Read the model definition and answer for the solid it produces. Units are mm, in the model's axes. Face numbers are marked on the shaded views. A direction names the side the tool comes from. Round coordinates to 2 decimals unless told otherwise and drop trailing zeros. Write each loop counter-clockwise with the first axis right and the second up, starting at its lowest first coordinate (ties: lowest second). Pieces come first, ordered by that corner, then holes. Notation, with made-up numbers: (73.5, -27.5) - (129.5, -27.5) arc R31 cw to (129.5, 0.5) - close; hole circle Ø9 at (29, 50). An arc over 180 degrees is marked (long way). One line per item, written item: value. Start each with the question number.
(1) A cutting plane is placed at A-A, the plane y = 3.5. Determine the outline of the cut face in (x, z), plus the area to 3 significant figures.
(2) For the marked faces 1 and 2, determine the directions among +Z, -Z, +X, -X, +Y, -Y from which every point of the face is accessible in a straight line to the end or side of a thin tool.
(3) Find the intervals of material crossed by L1, parallel to Y at x = 0, z = 0.85; L2, parallel to X at y = -3.5, z = 0.4; L3, parallel to Y at x = 10.25, z = 1.8, in increasing order.
(4) A cutting plane is placed at C-C, the plane y = -3.5. Determine the outline of the cut face in (x, z), plus the area to 3 significant figures.
(5) A cutting plane is placed at D-D, the plane z = 0.85. Determine the outline of the cut face in (x, y).
(6) Flat-ended cylindrical pins translate along their axes: pin 1 Ø1.8 at (x, y) = (7, 3.5) entering from -Z; pin 2 Ø1.5 at (x, y) = (6, 4.5) entering from +Z. Find the tip coordinate at first contact, or state that the pin passes through.
(7) A cutting plane is placed at B-B, the plane x = 0. Determine the outline of the cut face in (y, z).
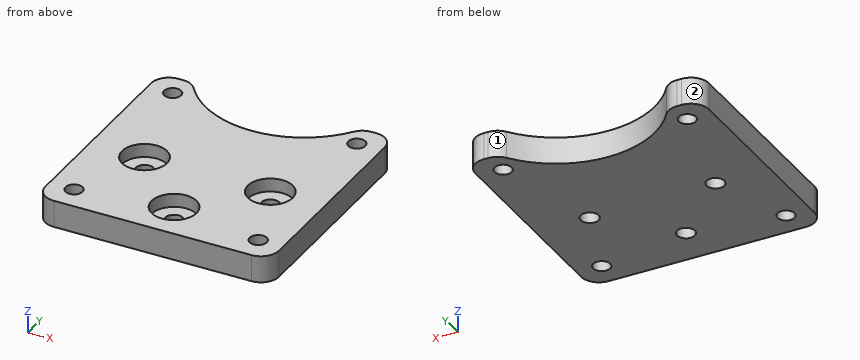
from build123d import *

# Parameters (mm, degrees)
SKETCH_1_R          = 1
SKETCH_1_R_2        = 0.95
EXTRUDE_1_DEPTH     = 3
SKETCH_2_R          = 2.5
CUT_EXTRUDE_1_DEPTH = 1.5
FILLET_1_R          = 2


with BuildPart() as part:
    # 草图1 → 凸台-拉伸1 (new body)
    with BuildSketch(Plane.XY):
        with BuildLine():
            Line((-13, -8), (13, -8))
            Line((13, -8), (13, 18.190012112))
            Line((13, 18.190012112), (9.43808773, 18.190012112))
            ThreePointArc((9.43808773, 18.190012112), (0, 12.840012112), (-9.43808773, 18.190012112))
            Line((-9.43808773, 18.190012112), (-13, 18.190012112))
            Line((-13, 18.190012112), (-13, -8))
        make_face()
        with Locations((7, 3.5)):
            Circle(SKETCH_1_R, mode=Mode.SUBTRACT)
        with Locations(Location((-7, 3.5, 0), (0, 0, 180))):
            Circle(SKETCH_1_R, mode=Mode.SUBTRACT)
        with Locations((0, -3.5)):
            Circle(SKETCH_1_R, mode=Mode.SUBTRACT)
        with Locations((10.25, 15.540012112)):
            Circle(SKETCH_1_R_2, mode=Mode.SUBTRACT)
        with Locations(Location((-10.25, 15.540012112, 0), (0, 0, 180))):
            Circle(SKETCH_1_R_2, mode=Mode.SUBTRACT)
        with Locations((-10.25, -5.159987888)):
            Circle(SKETCH_1_R_2, mode=Mode.SUBTRACT)
        with Locations(Location((10.25, -5.159987888, 0), (0, 0, 180))):
            Circle(SKETCH_1_R_2, mode=Mode.SUBTRACT)
    extrude(amount=EXTRUDE_1_DEPTH)

    # 草图2 → 切除-拉伸1 (cut)
    with BuildSketch(Plane.XY.offset(3)):
        with Locations((-7, 3.5)):
            Circle(SKETCH_2_R)
        with Locations((7, 3.5)):
            Circle(SKETCH_2_R)
        with Locations((0, -3.5)):
            Circle(SKETCH_2_R)
    extrude(amount=-CUT_EXTRUDE_1_DEPTH, mode=Mode.SUBTRACT)

    # 圆角1
    fillet_1_edges = [part.edges().sort_by_distance(p)[0] for p in [
        (13, -8, 1.5),
        (-13, -8, 1.5),
        (-13, 18.190012112, 1.5),
        (-9.43808773, 18.190012112, 1.5),
        (9.43808773, 18.190012112, 1.5),
        (13, 18.190012112, 1.5),
    ]]
    fillet(fillet_1_edges, radius=FILLET_1_R)


solid = part.part
Here are the results:
1. outline: (-13, 0) - (-8, 0) - (-8, 1.5) - (-9.5, 1.5) - (-9.5, 3) - (-13, 3) - close; (-6, 0) - (6, 0) - (6, 1.5) - (4.5, 1.5) - (4.5, 3) - (-4.5, 3) - (-4.5, 1.5) - (-6, 1.5) - close; (8, 0) - (13, 0) - (13, 3) - (9.5, 3) - (9.5, 1.5) - (8, 1.5) - close
1. area: 57.0 mm²
2. face 1: +Z, -Z, +Y
2. face 2: +Z, -Z, -X, +Y
3. L1: -8 to -4.5, -2.5 to 12.84
3. L2: -13 to -1, 1 to 13
3. L3: -8 to -6.11, -4.21 to 14.59, 16.49 to 18.17
4. outline: (-13, 0) - (-1, 0) - (-1, 1.5) - (-2.5, 1.5) - (-2.5, 3) - (-13, 3) - close; (1, 0) - (13, 0) - (13, 3) - (2.5, 3) - (2.5, 1.5) - (1, 1.5) - close
4. area: 67.5 mm²
5. outline: (-13, -6) arc R2 ccw to (-11, -8) - (11, -8) arc R2 ccw to (13, -6) - (13, 16.19) arc R2 ccw to (11, 18.19) - (10.51, 18.19) arc R2 ccw to (8.89, 17.37) arc R11 cw to (-8.89, 17.37) arc R2 ccw to (-10.51, 18.19) - (-11, 18.19) arc R2 ccw to (-13, 16.19) - close; hole circle Ø1.9 at (-10.25, -5.16); hole circle Ø1.9 at (-10.25, 15.54); hole circle Ø2 at (-7, 3.5); hole circle Ø2 at (0, -3.5); hole circle Ø2 at (7, 3.5); hole circle Ø1.9 at (10.25, -5.16); hole circle Ø1.9 at (10.25, 15.54)
6. pin 1: through
6. pin 2: z = 1.5
7. outline: (-8, 0) - (-4.5, 0) - (-4.5, 1.5) - (-6, 1.5) - (-6, 3) - (-8, 3) - close; (-2.5, 0) - (12.84, 0) - (12.84, 3) - (-1, 3) - (-1, 1.5) - (-2.5, 1.5) - close
